Read the model definition and answer for the solid it produces. Units are mm, in the model's axes. A direction names the side the tool comes from. Coordinates: 2 decimals unless noted, no trailing zeros. Loops run counter-clockwise (first coordinate to the right, second up) from the corner with the lowest first, then second, coordinate; pieces in that order, holes last. Notation, with made-up numbers: M -29.5,11 L 7.5,11 A10 ccw 7.5,16 Z; hole C 80.25,-38.5 d8. An arc over 180 degrees is marked long. One line per item, written item: value. Start each with the question number.
```python
from build123d import *

# Parameters (mm, degrees)
F0_R     = 1.5
F0_R_2   = 15.1
F0_R_3   = 2
F1_DEPTH = 8
F2_SIZE  = 16


with BuildPart() as f1:
    # F0 (on Top) → F1 (new body)
    with BuildSketch(Plane.XY):
        Polygon((32.5, -21), (32.5, 21), (-32.5, 21), (-32.5, -21), (-32.5, -36), (7.5, -36), (7.5, -21), align=None)
        with Locations((-28.763456, -31.263456)):
            Circle(F0_R, mode=Mode.SUBTRACT)
        with Locations((-12.5, -15)):
            Circle(F0_R_2, mode=Mode.SUBTRACT)
        with Locations((3.763456, -31.263456)):
            Circle(F0_R, mode=Mode.SUBTRACT)
        with Locations((25.5, -16)):
            Circle(F0_R_3, mode=Mode.SUBTRACT)
        with Locations((-28.763456, 1.263456)):
            Circle(F0_R, mode=Mode.SUBTRACT)
        with Locations((3.763456, 1.263456)):
            Circle(F0_R, mode=Mode.SUBTRACT)
        with Locations((25.5, 16)):
            Circle(F0_R_3, mode=Mode.SUBTRACT)
    extrude(amount=F1_DEPTH)

    # F2
    f2_edges = [f1.edges().sort_by_distance(p)[0] for p in [
        (-32.5, 21, 4),
    ]]
    chamfer(f2_edges, length=F2_SIZE)


solid = f1.part
```
1) For a pull along X with two mould halves and no side action, classify faces 3 (the face through (25.24, -14.017, 3.944)), 4 (the face through (3.44, -32.73, 3.94)), 5 (the face through (-32.5, -15, 4)), 6 (the face through (32.5, 0, 4)) as released by +X, released by -X, zero draft, split by the parting line, or undercut.
2) Section A-A (y = 16) is taken. Determine the outline of the cut face in (x, z).
3) A tool of negligible diameter and unlimited length cuts with its end or side. For faces 1 (the face through (25.24, 17.983, 3.944)), 2 (the face through (20, -21, 4)), from which of +Z, -Z, +X, -X, +Y, -Y can it reach the whole face along a straight path? Write none if from no direction.
4) Flat-ended cylindrical pins translate along their axes: pin 1 (6.5 mm diameter, centred on x = 25.5, y = -16, fed in from -Z); pin 2 (4 mm diameter, centred on x = 20, z = 6, fed in from -Y); pin 3 (2.5 mm diameter, centred on y = -25.5, z = 3.5, fed in from +X). Find the tip coordinate at first contact, or state that the pin passes through.
5) Section B-B (x = 25.5) is taken. Determine the outline of the cut face in (y, z).
6) Section C-C (x = -12.5) is taken. Determine the outline of the cut face in (y, z).
7) Section D-D (z = 2.25) is taken. Determine the outline of the cut face in (x, y), then the cut area to 3 significant figures.
8) Consider line 1 along Y through (x, z) = (25.5, 2); line 2 along Y through (x, z) = (-12.5, 5.75); line 3 along Y through (x, z) = (29.5, 2). Determine where each line is inside the solid, lowest interval first.
Results found:
1. face 3: undercut
1. face 4: undercut
1. face 5: released by -X
1. face 6: released by +X
2. outline: M -21.5,0 L 23.5,0 L 23.5,8 L -21.5,8 Z; M 27.5,0 L 32.5,0 L 32.5,8 L 27.5,8 Z
3. face 1: +Z, -Z
3. face 2: +Z, -Z, +X, -Y
4. pin 1: stops at z = 0
4. pin 2: stops at y = -21
4. pin 3: stops at x = 7.5
5. outline: M -21,0 L -18,0 L -18,8 L -21,8 Z; M -14,0 L 14,0 L 14,8 L -14,8 Z; M 18,0 L 21,0 L 21,8 L 18,8 Z
6. outline: M -36,0 L -30.1,0 L -30.1,8 L -36,8 Z; M 0.1,0 L 21,0 L 21,8 L 0.1,8 Z
7. outline: M -32.5,-36 L 7.5,-36 L 7.5,-21 L 32.5,-21 L 32.5,21 L -16.5,21 L -32.5,5 Z; hole C -28.76,-31.26 d3; hole C -28.76,1.26 d3; hole C -12.5,-15 d30.2; hole C 3.76,-31.26 d3; hole C 3.76,1.26 d3; hole C 25.5,-16 d4; hole C 25.5,16 d4
7. area: 2,430 mm²
8. line 1: y = -21 to -18, -14 to 14, 18 to 21
8. line 2: y = -36 to -30.1, 0.1 to 21
8. line 3: y = -21 to 21
